Read the model definition and answer for the solid it produces. Units are mm, in the model's axes. A direction names the side the tool comes from. Coordinates: 2 decimals unless noted, no trailing zeros. Write each loop counter-clockwise with the first axis right and the second up, starting at its lowest first coordinate (ties: lowest second). Pieces come first, ordered by that corner, then holes. Notation, with made-up numbers: (-1, 9.5) -> (6, 9.5) arc R22 cw to (6, 29.5) -> close; hole circle Ø1 at (45, -5). An arc over 180 degrees is marked (long way). Use CSV: the item, a comma, the result in double quotes.
from build123d import *

# Parameters (mm, degrees)
BOSS_EXTRUDE1_DEPTH           = 55
BOSS_EXTRUDE4_DEPTH           = 10
BOSS_EXTRUDE3_DEPTH           = 5
CSK_FOR_M4_SFHCS2_D           = 4.5
CSK_FOR_M4_SFHCS2_CSINK_D     = 8.96
CSK_FOR_M4_SFHCS2_CSINK_ANGLE = 90
FILLET4_R                     = 5
SKETCH12_R                    = 23.75
CUT_EXTRUDE2_DEPTH            = 33.05


with BuildPart() as part:
    # Sketch2 → Boss-Extrude1 (new body)
    with BuildSketch(Plane.XY):
        Polygon((-92.5, 34), (92.5, 34), (92.5, 0), (35, 0), (35, -15), (-35, -15), (-35, 0), (-92.5, 0), align=None)
    extrude(amount=BOSS_EXTRUDE1_DEPTH)

    # Sketch4 → Boss-Extrude4 (add)
    with BuildSketch(Plane.XY.offset(55)):
        with BuildLine():
            Line((-26.525, 4.65), (-3.725, 4.65))
            ThreePointArc((-3.725, 4.65), (-2.375, 3.3), (-3.725, 1.95))
            Line((-3.725, 1.95), (-26.525, 1.95))
            ThreePointArc((-26.525, 1.95), (-27.875, 3.3), (-26.525, 4.65))
        make_face()
        with BuildLine():
            Line((26.525, 1.95), (3.725, 1.95))
            ThreePointArc((3.725, 1.95), (2.375, 3.3), (3.725, 4.65))
            Line((3.725, 4.65), (26.525, 4.65))
            ThreePointArc((26.525, 4.65), (27.875, 3.3), (26.525, 1.95))
        make_face()
    extrude(amount=BOSS_EXTRUDE4_DEPTH)

    # Sketch6 → Boss-Extrude3 (add)
    with BuildSketch(Plane(origin=(0, 0, 0), x_dir=(-1, 0, 0), z_dir=(0, 0, -1))):
        with BuildLine():
            Line((-11.45, 25.475), (11.45, 25.475))
            ThreePointArc((11.45, 25.475), (12.75, 24.175), (11.45, 22.875))
            Line((11.45, 22.875), (-11.45, 22.875))
            ThreePointArc((-11.45, 22.875), (-12.75, 24.175), (-11.45, 25.475))
        make_face()
        with BuildLine():
            Line((16.8, 25.475), (42.2, 25.475))
            ThreePointArc((42.2, 25.475), (43.5, 24.175), (42.2, 22.875))
            Line((42.2, 22.875), (16.8, 22.875))
            ThreePointArc((16.8, 22.875), (15.5, 24.175), (16.8, 25.475))
        make_face()
        with BuildLine():
            Line((-16.8, 22.875), (-42.2, 22.875))
            ThreePointArc((-42.2, 22.875), (-43.5, 24.175), (-42.2, 25.475))
            Line((-42.2, 25.475), (-16.8, 25.475))
            ThreePointArc((-16.8, 25.475), (-15.5, 24.175), (-16.8, 22.875))
        make_face()
        with BuildLine():
            Line((-32.2, 7), (32.2, 7))
            ThreePointArc((32.2, 7), (35, 4.2), (32.2, 1.4))
            Line((32.2, 1.4), (-32.2, 1.4))
            ThreePointArc((-32.2, 1.4), (-35, 4.2), (-32.2, 7))
        make_face()
    extrude(amount=BOSS_EXTRUDE3_DEPTH)

    # CSK for M4 SFHCS2 (through all)
    with Locations(Plane.XZ):
        with Locations((-83.75, 11), (-83.75, 43), (-55.25, 43), (55.25, 43), (83.75, 43), (83.75, 11), (55.25, 11), (-55.25, 11)):
            CounterSinkHole(CSK_FOR_M4_SFHCS2_D / 2, CSK_FOR_M4_SFHCS2_CSINK_D / 2, counter_sink_angle=CSK_FOR_M4_SFHCS2_CSINK_ANGLE)

    # Fillet4
    fillet4_edges = [part.edges().sort_by_distance(p)[0] for p in [
        (-92.5, 34, 27.5),
        (92.5, 34, 27.5),
        (92.5, 17, 55),
        (0, 34, 55),
        (-92.5, 17, 55),
        (-92.5, 17, 0),
        (0, 34, 0),
        (92.5, 17, 0),
    ]]
    fillet(fillet4_edges, radius=FILLET4_R)

    # Sketch12 → Cut-Extrude2 (cut, through all)
    with BuildSketch(Plane.XZ.offset(-1.95)):
        with Locations((0, 80.5)):
            Circle(SKETCH12_R)
    extrude(amount=-CUT_EXTRUDE2_DEPTH, mode=Mode.SUBTRACT)


solid = part.part
1. A cutting plane is placed at B-B (x = -38.5). Give the vertices of the cut face in (y, z) (3 decimals), and give its area (3 significant figures).
Solutions:
outline,"(0, 0) -> (22.875, 0) -> (22.875, -5) -> (25.475, -5) -> (25.475, 0) -> (29, 0) arc R5 ccw to (34, 5) -> (34, 50) arc R5 ccw to (29, 55) -> (0, 55) -> close"
area,"1,870 mm^2"
2. A cutting plane is placed at A-A (z = 43). Give the number of separate pieces and of enclosed holes in the cut face, and give its area (3 significant figures).
Solutions:
separate pieces,"5"
enclosed holes,"0"
area,"6,700 mm^2"
3. For a pull along X with two mould halves and no side action, classify faces 4 (the flat face through (29, 22.875, -2)), 5 (the conical face through (53, 2.12, 11.71)), 6 (the cylindrical face through (-91, 14.7, 53.57)) as pulls with the +X half, pulls with the -X half, needs draft (parallel to the pull), parting line crosses it, or undercut.
Solutions:
face 4,"needs draft"
face 5,"undercut"
face 6,"pulls with the -X half"
4. A tool of negligible diameter and unlimited length cuts with its end or side. For faces 1 (the flat face through (18, 1.95, 59)), 2 (the flat face through (-63, 0, 27)), 3 (the flat face through (64, 0, 27)), from which of +Z, -Z, +X, -X, +Y, -Y can it reach the whole face along a straight path? Write none if from no direction.
Solutions:
face 1,"+Z, +X, -X, -Y"
face 2,"+Z, -Z, -X, -Y"
face 3,"+Z, -Z, +X, -Y"
5. A cutting plane is placed at C-C (z = 23). Give the vertices of the cut face in (x, y), and give its area (3 significant figures).
Solutions:
outline,"(-92.5, 0) -> (-35, 0) -> (-35, -15) -> (35, -15) -> (35, 0) -> (92.5, 0) -> (92.5, 29) arc R5 ccw to (87.5, 34) -> (-87.5, 34) arc R5 ccw to (-92.5, 29) -> close"
area,"7,330 mm^2"
6. A cutting plane is placed at D-D (y = -11). Give the vertices of the cut face in (x, z), and give its area (3 significant figures).
Solutions:
outline,"(-35, 0) -> (35, 0) -> (35, 55) -> (-35, 55) -> close"
area,"3,850 mm^2"
7. Each of these flat-tipped pins is pushed along its axis until it touches: pin 1 Ø10 at (y, z) = (-6.5, 16) entering from +X; pin 2 Ø5.5 at (x, z) = (-30.5, -3.5) entering from -Y; pin 3 Ø5 at (x, z) = (-11, 62) entering from +Y. Where does it stop, or does it pass through?
Solutions:
pin 1,"stops at x = 35"
pin 2,"stops at y = 1.4"
pin 3,"stops at y = 4.65"
8. Find the intervals of material crossed by line 1 along X through (y, z) = (26, 43); line 2 along Z through (x, y) = (-55.25, 11); line 3 along X through (y, z) = (-11, 41), in increasing order.
Solutions:
line 1,"x = -92.5 to -86, -81.5 to -57.5, -53 to 53, 57.5 to 81.5, 86 to 92.5"
line 2,"z = 0 to 8.75, 13.25 to 40.75, 45.25 to 55"
line 3,"x = -35 to 35"
